```python
from build123d import *

# Parameters (mm, degrees)
F1_DEPTH = 1.5875


with BuildPart() as f1:
    # F0 (on Right) → F1 (new body, symmetric)
    with BuildSketch(Plane.YZ):
        with BuildLine():
            ThreePointArc((0, -3.175), (-2.2450640303, -2.2450640303), (-3.175, 0))
            Line((-3.175, 0), (-45.8724, 0))
            Line((-45.8724, 0), (-45.8724, -13.462))
            ThreePointArc((-45.8724, -13.462), (-45.6738112484, -13.4645046841), (-45.4753488371, -13.4720171431))
            Line((-45.4753488371, -13.4720171431), (-0.7941023258, -15.7279657139))
            ThreePointArc((-0.7941023258, -15.7279657139), (-0.3971775033, -15.7429906317), (0, -15.748))
            Line((0, -15.748), (0, -3.175))
        make_face()
        with BuildLine():
            ThreePointArc((51.83759, -10.8726027699), (58.8815419933, -7.3470240921), (61.722, 0))
            Line((61.722, 0), (53.975, 0))
            ThreePointArc((53.975, 0), (53.0450640303, -2.2450640303), (50.8, -3.175))
            ThreePointArc((50.8, -3.175), (48.5549359697, -2.2450640303), (47.625, 0))
            Line((47.625, 0), (36.5252, 0))
            Line((36.5252, 0), (3.175, 0))
            ThreePointArc((3.175, 0), (2.2450640303, -2.2450640303), (0, -3.175))
            Line((0, -3.175), (0, -15.748))
            ThreePointArc((0, -15.748), (0.7488772211, -15.7301839439), (1.49606, -15.6767760868))
            Line((1.49606, -15.6767760868), (51.83759, -10.8726027699))
        make_face()
        with BuildLine():
            Line((51.83759, 10.8726027699), (1.49606, 15.6767760868))
            ThreePointArc((1.49606, 15.6767760868), (0.7488772211, 15.7301839439), (0, 15.748))
            Line((0, 15.748), (0, 3.175))
            ThreePointArc((0, 3.175), (2.2450640303, 2.2450640303), (3.175, 0))
            Line((3.175, 0), (36.5252, 0))
            Line((36.5252, 0), (47.625, 0))
            ThreePointArc((47.625, 0), (48.5549359697, 2.2450640303), (50.8, 3.175))
            ThreePointArc((50.8, 3.175), (53.0450640303, 2.2450640303), (53.975, 0))
            Line((53.975, 0), (61.722, 0))
            ThreePointArc((61.722, 0), (58.8815419933, 7.3470240921), (51.83759, 10.8726027699))
        make_face()
        with BuildLine():
            ThreePointArc((39.7002, 3.175), (38.7702640303, 0.9299359697), (36.5252, 0))
            ThreePointArc((36.5252, 0), (34.2801359697, 0.9299359697), (33.3502, 3.175))
            ThreePointArc((33.3502, 3.175), (34.2801359697, 5.4200640303), (36.5252, 6.35))
            ThreePointArc((36.5252, 6.35), (38.7702640303, 5.4200640303), (39.7002, 3.175))
        make_face(mode=Mode.SUBTRACT)
        with BuildLine():
            Line((0, 3.175), (0, 15.748))
            ThreePointArc((0, 15.748), (-0.5672962051, 15.7377787192), (-1.133856, 15.7071281452))
            Line((-1.133856, 15.7071281452), (-45.8724, 12.4775710883))
            Line((-45.8724, 12.4775710883), (-45.8724, 0))
            Line((-45.8724, 0), (-3.175, 0))
            ThreePointArc((-3.175, 0), (-2.2450640303, 2.2450640303), (0, 3.175))
        make_face()
        with BuildLine():
            Line((-45.8724, 0), (-45.8724, 12.4775710883))
            Line((-45.8724, 12.4775710883), (-63.5, 11.2050813091))
            Line((-63.5, 11.2050813091), (-63.5, 11.176))
            Line((-63.5, 11.176), (-63.5, 3.175))
            ThreePointArc((-63.5, 3.175), (-61.2549359697, 2.2450640303), (-60.325, 0))
            Line((-60.325, 0), (-45.8724, 0))
        make_face()
        with BuildLine():
            Line((-45.8724, -13.462), (-45.8724, 0))
            Line((-45.8724, 0), (-60.325, 0))
            ThreePointArc((-60.325, 0), (-61.2549359697, -2.2450640303), (-63.5, -3.175))
            Line((-63.5, -3.175), (-63.5, -21.336))
            Line((-63.5, -21.336), (-53.7779584797, -21.336))
            Line((-53.7779584797, -21.336), (-53.7149674997, -20.6331408299))
            ThreePointArc((-53.7149674997, -20.6331408299), (-51.1858528743, -15.5250539021), (-45.8724, -13.462))
        make_face()
        with BuildLine():
            Line((-63.5, -21.336), (-63.5, -3.175))
            ThreePointArc((-63.5, -3.175), (-65.7450640303, -2.2450640303), (-66.675, 0))
            Line((-66.675, 0), (-74.676, 0))
            ThreePointArc((-74.676, 0), (-74.6670412581, -0.4473986372), (-74.640179395, -0.89408))
            Line((-74.640179395, -0.89408), (-72.9995674098, -21.336))
            Line((-72.9995674098, -21.336), (-63.5, -21.336))
        make_face()
        with BuildLine():
            Line((-63.5, 3.175), (-63.5, 11.176))
            ThreePointArc((-63.5, 11.176), (-63.9025973068, 11.1687461878), (-64.304672, 11.1469941676))
            ThreePointArc((-64.304672, 11.1469941676), (-71.6821754525, 7.612816881), (-74.676, 0))
            Line((-74.676, 0), (-66.675, 0))
            ThreePointArc((-66.675, 0), (-65.7450640303, 2.2450640303), (-63.5, 3.175))
        make_face()
        with BuildLine():
            Line((-53.7779584797, -21.336), (-63.5, -21.336))
            Line((-63.5, -21.336), (-63.5, -41.275))
            ThreePointArc((-63.5, -41.275), (-61.2549359697, -42.2049359697), (-60.325, -44.45))
            Line((-60.325, -44.45), (-55.8494595357, -44.45))
            Line((-55.8494595357, -44.45), (-53.7779584797, -21.336))
        make_face()
        with BuildLine():
            Line((-63.5, -41.275), (-63.5, -21.336))
            Line((-63.5, -21.336), (-72.9995674098, -21.336))
            Line((-72.9995674098, -21.336), (-71.1445016709, -44.45))
            Line((-71.1445016709, -44.45), (-66.675, -44.45))
            ThreePointArc((-66.675, -44.45), (-65.7450640303, -42.2049359697), (-63.5, -41.275))
        make_face()
        with BuildLine():
            Line((-55.9104185487, -45.1301862936), (-55.8494595357, -44.45))
            Line((-55.8494595357, -44.45), (-60.325, -44.45))
            ThreePointArc((-60.325, -44.45), (-61.2549359697, -46.6950640303), (-63.5, -47.625))
            Line((-63.5, -47.625), (-63.5, -52.07))
            ThreePointArc((-63.5, -52.07), (-58.3579488313, -50.0734962238), (-55.9104185487, -45.1301862936))
        make_face()
        with BuildLine():
            ThreePointArc((-63.5, -47.625), (-65.7450640303, -46.6950640303), (-66.675, -44.45))
            Line((-66.675, -44.45), (-71.1445016709, -44.45))
            Line((-71.1445016709, -44.45), (-71.0955768603, -45.0596))
            ThreePointArc((-71.0955768603, -45.0596), (-68.6681354471, -50.049533552), (-63.5, -52.07))
            Line((-63.5, -52.07), (-63.5, -47.625))
        make_face()
    extrude(amount=F1_DEPTH, both=True)


solid = f1.part
```
Work out the finished part from the listing and answer in its coordinate system (mm). Round coordinates to 2 decimals unless told otherwise and drop trailing zeros. Write each loop counter-clockwise with the first axis right and the second up, starting at its lowest first coordinate (ties: lowest second). Pieces come first, ordered by that corner, then holes. Notation, with made-up numbers: (84.5, 66.25) -> (88.5, 66.25) arc R26 ccw to (88.5, 91.25) -> close; hole circle Ø3 at (31.25, 37). An arc over 180 degrees is marked (long way). Write each question's results on one line, items separated by ' | '.
Q1. A flat-ended cylindrical pin translates along its axis: P1, Ø1.5, axis at x = 0.5, y = 8, coming from the +Z side. Find the tip coordinate at first contact, or state that the pin passes through.
Data:
P1: z = 15.13
Q2. Section C-C, the plane y = -13 is taken. Write down the section's boundary in (x, z).
Data:
outline: (-1.59, -15.11) -> (1.59, -15.11) -> (1.59, 14.85) -> (-1.59, 14.85) -> close
Q3. Section B-B, the plane x = 1.05 is taken. Give the number of separate pieces and of enclosed holes in the cut face, then the cut area to 3 significant figures.
Data:
separate pieces: 1 | enclosed holes: 5 | area: 4,050 mm^2
Q4. Section D-D, the plane z = -26 is taken. Write down the section's boundary in (x, y).
Data:
outline: (-1.59, -72.63) -> (1.59, -72.63) -> (1.59, -54.2) -> (-1.59, -54.2) -> close
Q5. Straight lines are drawn through the part: line 1 along Y through (x, z) = (-1.15, -45); line 2 along Z through (x, y) = (-0.65, -1); line 3 along Y through (x, z) = (0.7, -42). For each, find the intervals that lie inside material, in ascending order. Write a range as [from, to].
Data:
line 1: [-71.1, -66.63], [-60.37, -55.9] | line 2: [-15.72, -3.01], [3.01, 15.72] | line 3: [-71.34, -65.52], [-61.48, -55.63]
Q6. Section A-A, the plane z = 4.5 is taken. Write down the section's boundary in (x, y).
Data:
outline: (-1.59, -73.73) -> (1.59, -73.73) -> (1.59, 33.64) -> (-1.59, 33.64) -> close; (-1.59, 39.41) -> (1.59, 39.41) -> (1.59, 60.75) -> (-1.59, 60.75) -> close
